Geometry check sheet. Reference: the model listing, model coordinates, mm. Face numbers are marked on the shaded views. A direction names the side the tool comes from. Coordinates: 2 decimals unless noted, no trailing zeros. Write each loop counter-clockwise with the first axis right and the second up, starting at its lowest first coordinate (ties: lowest second). Pieces come first, ordered by that corner, then holes. Notation, with made-up numbers: M -39,44.25 L 2,44.25 A32 cw 2,78.25 Z; hole C -19.5,-18 d6. An arc over 180 degrees is marked long. Write each question's results on one line, items separated by ' | '.
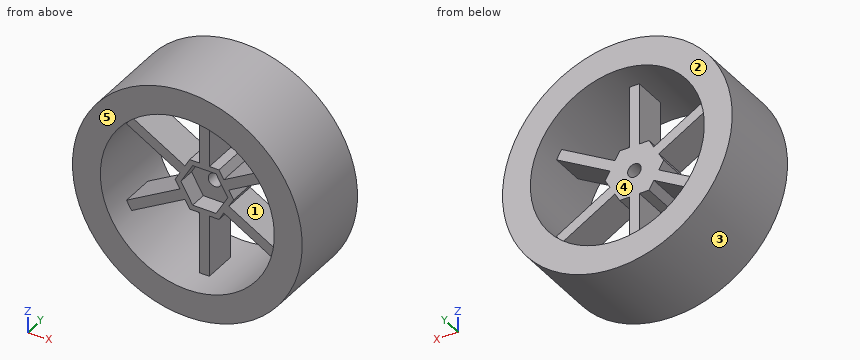
```python
from build123d import *

# Parameters (mm, degrees)
SKETCH_1_R      = 34
SKETCH_1_R_2    = 25.75
EXTRUDE_1_DEPTH = 26
EXTRUDE_2_DEPTH = 5
SKETCH_2_4_R    = 2
EXTRUDE_3_DEPTH = 5


with BuildPart() as part:
    # Sketch 1 → Extrude 1 (new body)
    with BuildSketch(Plane(origin=(0, 0, 0), x_dir=(1, 0, 0), z_dir=(0, 1, 0))):
        with Locations(Location((0, 0, 0), (0, 0, 90))):
            Circle(SKETCH_1_R)
        with Locations(Location((0, 0, 0), (0, 0, 90))):
            Circle(SKETCH_1_R_2, mode=Mode.SUBTRACT)
    extrude(amount=EXTRUDE_1_DEPTH)

    # Sketch 2 → Extrude 2 (add, symmetric)
    # profile 1 of 7: a face of its own
    with BuildSketch(Plane(origin=(0, 13, 0), x_dir=(1, 0, 0), z_dir=(0, 1, 0))):
        with BuildLine():
            Line((5.745190528, 5.049038106), (7.245190528, 2.450961894))
            Line((7.245190528, 2.450961894), (23.012285934, 11.554098671))
            ThreePointArc((23.012285934, 11.554098671), (22.300154147, 12.875), (21.512285934, 14.152174882))
            Line((21.512285934, 14.152174882), (5.745190528, 5.049038106))
        make_face()
    # profile 2 of 7: a face of its own
    with BuildSketch(Plane(origin=(0, 13, 0), x_dir=(1, 0, 0), z_dir=(0, 1, 0))):
        with BuildLine():
            Line((23.012285934, -11.554098671), (7.245190528, -2.450961894))
            Line((7.245190528, -2.450961894), (5.745190528, -5.049038106))
            Line((5.745190528, -5.049038106), (21.512285934, -14.152174882))
            ThreePointArc((21.512285934, -14.152174882), (22.300154147, -12.875), (23.012285934, -11.554098671))
        make_face()
    # profile 3 of 7: a face of its own
    with BuildSketch(Plane(origin=(0, 13, 0), x_dir=(1, 0, 0), z_dir=(0, 1, 0))):
        with BuildLine():
            Line((1.5, -25.706273553), (1.5, -7.5))
            Line((1.5, -7.5), (-1.5, -7.5))
            Line((-1.5, -7.5), (-1.5, -25.706273553))
            ThreePointArc((-1.5, -25.706273553), (0, -25.75), (1.5, -25.706273553))
        make_face()
    # profile 4 of 7: a face of its own
    with BuildSketch(Plane(origin=(0, 13, 0), x_dir=(1, 0, 0), z_dir=(0, 1, 0))):
        with BuildLine():
            ThreePointArc((-23.012285934, -11.554098671), (-22.300154147, -12.875), (-21.512285934, -14.152174882))
            Line((-21.512285934, -14.152174882), (-5.745190528, -5.049038106))
            Line((-5.745190528, -5.049038106), (-7.245190528, -2.450961894))
            Line((-7.245190528, -2.450961894), (-23.012285934, -11.554098671))
        make_face()
    # profile 5 of 7: a face of its own
    with BuildSketch(Plane(origin=(0, 13, 0), x_dir=(1, 0, 0), z_dir=(0, 1, 0))):
        with BuildLine():
            Line((-5.745190528, 5.049038106), (-21.512285934, 14.152174882))
            ThreePointArc((-21.512285934, 14.152174882), (-22.300154147, 12.875), (-23.012285934, 11.554098671))
            Line((-23.012285934, 11.554098671), (-7.245190528, 2.450961894))
            Line((-7.245190528, 2.450961894), (-5.745190528, 5.049038106))
        make_face()
    # profile 6 of 7: a face of its own
    with BuildSketch(Plane(origin=(0, 13, 0), x_dir=(1, 0, 0), z_dir=(0, 1, 0))):
        with BuildLine():
            Line((-1.5, 7.5), (1.5, 7.5))
            Line((1.5, 7.5), (1.5, 25.706273553))
            ThreePointArc((1.5, 25.706273553), (0, 25.75), (-1.5, 25.706273553))
            Line((-1.5, 25.706273553), (-1.5, 7.5))
        make_face()
    # profile 7 of 7: a face of its own
    with BuildSketch(Plane(origin=(0, 13, 0), x_dir=(1, 0, 0), z_dir=(0, 1, 0))):
        Polygon((-4.330127019, -7.5), (4.330127019, -7.5), (8.660254038, 0), (4.330127019, 7.5), (-4.330127019, 7.5), (-8.660254038, 0), align=None)
        Polygon((3.464101615, -6), (6.92820323, 0), (3.464101615, 6), (-3.464101615, 6), (-6.92820323, 0), (-3.464101615, -6), align=None, mode=Mode.SUBTRACT)
    extrude(amount=EXTRUDE_2_DEPTH, both=True)

    # Sketch 2_4 → Extrude 3 (add)
    with BuildSketch(Plane(origin=(0, 13, 0), x_dir=(1, 0, 0), z_dir=(0, 1, 0))):
        Polygon((3.464101615, -6), (6.92820323, 0), (3.464101615, 6), (-3.464101615, 6), (-6.92820323, 0), (-3.464101615, -6), align=None)
        with Locations(Location((0, 0, 0), (0, 0, 270))):
            Circle(SKETCH_2_4_R, mode=Mode.SUBTRACT)
    extrude(amount=EXTRUDE_3_DEPTH)


solid = part.part
```
Q1. Scan lines: probe 1 along X at (y, z) = (12, 0); probe 2 along X at (y, z) = (14.4, 0); probe 3 along Z at (x, y) = (13, 16.5). Record each from-to range of solid material in increasing order.
Geometry check:
probe 1: x = -34 to -25.75, -8.66 to -6.93, 6.93 to 8.66, 25.75 to 34 | probe 2: x = -34 to -25.75, -8.66 to -2, 2 to 8.66, 25.75 to 34 | probe 3: z = -31.42 to -22.23, -9.24 to -5.77, 5.77 to 9.24, 22.23 to 31.42
Q2. Sectioned sample at B-B on y = 15. Give the number of separate pieces and of enclosed holes in the cut face, and give its area (3 significant figures).
Geometry check:
separate pieces: 1 | enclosed holes: 7 | area: 2,060 mm2
Q3. Sectioned sample at C-C on z = 17.5. Record the cut outline in (x, y).
Geometry check:
outline: M -29.15,0 L -18.89,0 L -18.89,26 L -29.15,26 Z; M -1.5,8 L 1.5,8 L 1.5,18 L -1.5,18 Z; M 18.89,0 L 29.15,0 L 29.15,26 L 18.89,26 Z
Q4. Sectioned sample at A-A on x = 0. Record the cut outline in (y, z), and give its area (3 significant figures).
Geometry check:
outline: M 0,-34 L 26,-34 L 26,-25.75 L 18,-25.75 L 18,-2 L 13,-2 L 13,-6 L 8,-6 L 8,-25.75 L 0,-25.75 Z; M 0,25.75 L 8,25.75 L 8,6 L 13,6 L 13,2 L 18,2 L 18,25.75 L 26,25.75 L 26,34 L 0,34 Z | area: 864 mm2
Q5. Mould release check, pull along X, two halves, no side actions. Record for the marked faces 3, 4 and 5: pulls with the +X half, pulls with the -X half, needs draft (parallel to the pull), parting line crosses it, or undercut.
Geometry check:
face 3: parting line crosses it | face 4: undercut | face 5: needs draft
Q6. Depth check by flat-ended pin: P1, Ø0.8, axis at x = -3, y = 11, coming from the +Z side; P2, Ø2, axis at x = -18.5, y = 10, coming from the -Z side; P3, Ø5, axis at y = 14, z = -12.5, coming from the +X side; P4, Ø1.5, axis at x = -0.5, y = 11.5, coming from the +Z side. Enter the tip coordinate at first touch or a pass-through.
Geometry check:
P1: stops at z = 33.9 | P2: stops at z = -29.15 | P3: stops at x = 32.5 | P4: stops at z = 34
Q7. Sectioned sample at D-D on z = 8.5. Record the cut outline in (x, y).
Geometry check:
outline: M -32.92,0 L -24.31,0 L -24.31,26 L -32.92,26 Z; M -17.72,8 L -11.72,8 L -11.72,18 L -17.72,18 Z; M -1.5,8 L 1.5,8 L 1.5,18 L -1.5,18 Z; M 11.72,8 L 17.72,8 L 17.72,18 L 11.72,18 Z; M 24.31,0 L 32.92,0 L 32.92,26 L 24.31,26 Z
Q8. Access from +Z, -Z, +X, -X, +Y, -Y to the whole of each face (thin tool, end or side, straight path). Record for the marked faces 1 and 2.
Geometry check:
face 1: +Y, -Y | face 2: +Z, -Z, +X, -X, +Y
